from build123d import *

# Parameters (mm, degrees)
EXTRUDE_1_DEPTH = 60
SKETCH_1_3_R    = 9
SKETCH_1_3_R_2  = 8
EXTRUDE_2_DEPTH = 40


with BuildPart() as part:
    # Sketch 1 → Extrude 1 (new, symmetric)
    with BuildSketch(Plane.XY):
        with BuildLine():
            Line((2.783882181, 7.5), (-2.783882181, 7.5))
            ThreePointArc((-2.783882181, 7.5), (-4.567764363, -6.567764363), (8, 0))
            ThreePointArc((8, 0), (6.567764363, 4.567764363), (2.783882181, 7.5))
        make_face()
    extrude(amount=EXTRUDE_1_DEPTH, both=True)

    # Sketch 1_3 → Extrude 2 (add, symmetric)
    # profile 1 of 3: a face of its own
    with BuildSketch(Plane.XY):
        Circle(SKETCH_1_3_R)
        Circle(SKETCH_1_3_R_2, mode=Mode.SUBTRACT)
    # profile 2 of 3: a face of its own
    with BuildSketch(Plane.XY):
        with BuildLine():
            ThreePointArc((2.783882181, 7.5), (0, 8), (-2.783882181, 7.5))
            Line((-2.783882181, 7.5), (2.783882181, 7.5))
        make_face()
    # profile 3 of 3: a face of its own
    with BuildSketch(Plane.XY):
        with BuildLine():
            Line((2.783882181, 7.5), (-2.783882181, 7.5))
            ThreePointArc((-2.783882181, 7.5), (-4.567764363, -6.567764363), (8, 0))
            ThreePointArc((8, 0), (6.567764363, 4.567764363), (2.783882181, 7.5))
        make_face()
    extrude(amount=EXTRUDE_2_DEPTH, both=True)

    # Sketch 4 → Hole Wizard M6 _1 (revolve, cut)
    with BuildSketch(Plane(origin=(0, 0, 60), x_dir=(0, -1, 0), z_dir=(1, 0, 0))):
        Polygon((0, 0), (0, 19.502151548), (2.5, 18), (2.5, 0), align=None)
    hole_wizard_m6_1 = revolve(axis=Axis((0, 0, 66.35), (0, 0, -1)), mode=Mode.SUBTRACT)

    # Mirror 1: Hole Wizard M6 _1 across plane
    add(hole_wizard_m6_1.mirror(Plane.XY), mode=Mode.SUBTRACT)


solid = part.part
Verification items for the finished model (mm, model axes). A direction names the side the tool comes from. Round coordinates to 2 decimals unless told otherwise and drop trailing zeros. Order: outer loops, then holes, each group sorted by start corner. A loop starts at its lowest first (then second) coordinate and runs counter-clockwise, first axis right, second up. Notation, with made-up numbers: (54.25, -4.75) -> (110.25, -4.75) arc R25 ccw to (110.25, 30.25) -> close; hole circle Ø4 at (11, 57). An arc over 180 degrees is marked (long way). Put each result on its own line as item: value.
1) Set-up check for faces 4 (the flat face through (0, 7.5, 50)), 5 (the cylindrical face through (2.44, 0.54, -51.13)), 6 (the cylindrical face through (2.44, 0.54, 51.13)): record each of +Z, -Z, +X, -X, +Y, -Y from which the full face is reachable in a straight line by a thin tool's end or side.
Final values:
face 4: +Z, +X, -X, +Y
face 5: -Z
face 6: +Z
2) Section check B-B (x = 6.25). Record the cut outline in (y, z), then the cut area to 3 significant figures.
Final values:
outline: (-6.48, -40) -> (-4.99, -40) -> (-4.99, -60) -> (4.99, -60) -> (4.99, -40) -> (6.48, -40) -> (6.48, 40) -> (4.99, 40) -> (4.99, 60) -> (-4.99, 60) -> (-4.99, 40) -> (-6.48, 40) -> close
area: 1,440 mm^2
3) Section check A-A (y = 5.25). Record the cut outline in (x, z), then the cut area to 3 significant figures.
Final values:
outline: (-7.31, -40) -> (-6.04, -40) -> (-6.04, -60) -> (6.04, -60) -> (6.04, -40) -> (7.31, -40) -> (7.31, 40) -> (6.04, 40) -> (6.04, 60) -> (-6.04, 60) -> (-6.04, 40) -> (-7.31, 40) -> close
area: 1,650 mm^2
4) Section check D-D (z = -25). Record the cut outline in (x, y), then the cut area to 3 significant figures.
Final values:
outline: circle Ø18 at (0, 0)
area: 254 mm^2
5) Depth check by flat-ended pin: pin 1 (1.7 mm diameter, centred on x = -0.5, z = 51.5, fed in from +Y); pin 2 (3 mm diameter, centred on x = 0, y = 0, fed in from -Z); pin 3 (5 mm diameter, centred on x = -5, z = -44, fed in from -Y). Enter the tip coordinate at first touch or a pass-through.
Final values:
pin 1: stops at y = 7.5
pin 2: stops at z = -41.4
pin 3: stops at y = -7.6
6) Material ranges on line 1 (X direction, y = 0, z = 54); line 2 (Y direction, x = 0, z = -54.75); line 3 (Z direction, x = 7.5, y = -4.75), recorded low to high.
Final values:
line 1: x = -8 to -2.5, 2.5 to 8
line 2: y = -8 to -2.5, 2.5 to 7.5
line 3: z = -40 to 40
7) Section check C-C (z = 47.5). Record the cut outline in (x, y), then the cut area to 3 significant figures.
Final values:
outline: (-2.78, 7.5) arc R8 ccw (long way) to (2.78, 7.5) -> close; hole circle Ø5 at (0, 0)
area: 180 mm^2
8) Mould release check, pull along X, two halves, no side actions. Record for faces 1 (the flat face through (0, 7.5, -50)), 2 (the cylindrical face through (0, -8, -50)), 3 (the conical face through (0.424, 0.094, 40.759)): +X half, -X half, draft (parallel to the pull), parting line (faces both ways), or undercut.
Final values:
face 1: draft
face 2: parting line
face 3: undercut
